Source: CAD feature listing. Evaluate the final solid. Frame: model axes, mm. A direction names the side the tool comes from. Give positions to 0.01 mm unless a question says otherwise; leave off trailing zeros. Order: outer loops, then holes, each group sorted by start corner. A loop starts at its lowest first (then second) coordinate and runs counter-clockwise, first axis right, second up.
1) Section A-A, the plane x = 0. Return loops of the section in (y, z), plus the area to 3 significant figures.
2) Section B-B, the plane z = 5. Return loops of the section in (x, y).
3) Draft query along Y for faces 3 (the face through (15.035, 38.636, 2.958)), 4 (the face through (2, 14, 6)), 5 (the face through (0, 11.5, 3)), 6 (the face through (15, 40, 3)). Return one class per face: released by +Y, released by -Y, zero draft, split by the parting line, or undercut.
4) Material intervals for line 1 (Y direction, x = 1, z = 3.25); line 2 (X direction, y = 14.5, z = 3.25); line 3 (Y direction, x = 0, z = 4.75), sorted ascending.
5) First-contact query: P1, Ø2, axis at x = 6, z = 8, coming from the +Y side; P2, Ø1.5, axis at y = 27.5, z = 8.5, coming from the +X side; P3, Ø4, axis at x = 6, y = 23, coming from the -Z side; P4, Ø6, axis at x = -8.5, y = 17, coming from the -Z side. Flat tips, straight axial feed; report the tip coordinate or a pass-through.
6) Section D-D, the plane z = 1. Return loops of the section in (x, y), plus the area to 3 significant figures.
7) Access query for faces 1 (the face through (0, 35, 0)), 2 (the face through (13, 37, 6)). Directions: +Z, -Z, +X, -X, +Y, -Y. A direction counts if a zero-diameter tool reaches every point of the face in a straight line with its end or side. Return the directions, or none.
8) Section C-C, the plane y = 14.5. Return loops of the section in (x, z).
```python
from build123d import *
from build123d.topology import SkipClean

# Parameters (mm, degrees)
SKICA1_R                            = 1.650000859
SKICA1_R_2                          = 1.650000856
SKICA1_R_3                          = 1.649999795
P_IDAT_VYSUNUT_M1_DEPTH             = 2
P_IDAT_VYSUNUT_M3_REACH             = 52.341
P_IDAT_VYSUNUT_M3_DIRECTION_2_REACH = 52.341
SKICA3_R                            = 7.749999856
ODEBRAT_VYSUNUT_M1_DEPTH            = 50
SKICA5_W                            = 5.707521684
SKICA5_H                            = 11.749115372
SKICA5_W_2                          = 4.565648586
ODEBRAT_VYSUNUT_M2_DEPTH            = 100
SKICA6_W                            = 8.00000038
SKICA6_H                            = 6.259476141
SKICA6_R                            = 1.649999795
SKICA6_W_2                          = 7.999999449
SKICA6_H_2                          = 6.147887642
SKICA6_R_2                          = 1.650000859
SKICA6_R_3                          = 1.650000856
P_IDAT_VYSUNUT_M4_DEPTH             = 4


with BuildPart() as part:
    # Skica1 → Přidat vysunutím1 (new body)
    with BuildSketch(Plane.XY):
        Polygon((19.249999896, 35.500001162), (19.249999896, 33.428542316), (4.00000019, 16.00000076), (4.00000019, 11.500000022), (-4.00000019, 11.500000022), (-4.00000019, 16.00000076), (-19.249999896, 33.42806357), (-19.249999896, 35.500001162), (-19.249999896, 39.999999106), (-11.250000447, 39.999999106), (-11.250000447, 35.500001162), (11.250000447, 35.500001162), (11.250000447, 39.999999106), (19.249999896, 39.999999106), align=None)
        with Locations((-15.249999503, 37.000001471)):
            Circle(SKICA1_R, mode=Mode.SUBTRACT)
        with Locations((15.249998879, 37.000001475)):
            Circle(SKICA1_R_2, mode=Mode.SUBTRACT)
        with Locations((1.87e-07, 14.499999779)):
            Circle(SKICA1_R_3, mode=Mode.SUBTRACT)
    extrude(amount=P_IDAT_VYSUNUT_M1_DEPTH)

    # Přidat vysunutím3: up to this face of the body (flat: up to its plane)
    p_idat_vysunut_m3_end = Plane(part.part.faces().sort_by_distance((11.625000043, 24.714271538, 1))[0])
    # Skica2 → Přidat vysunutím3 (add, up to the picked face)
    with BuildSketch(Plane(origin=(-11.250000447, 0, 0), x_dir=(0, 0, -1), z_dir=(1, 0, 0)), mode=Mode.PRIVATE) as p_idat_vysunut_m3_sk1:
        with BuildLine():
            Line((-2, 35.453607186), (-2, 33.44155343))
            ThreePointArc((-2, 33.44155343), (-8.800000314, 25.749999709), (-2, 18.058445988))
            Line((-2, 18.058445988), (-2, 16.046392232))
            ThreePointArc((-2, 16.046392232), (-10.800000314, 25.749999709), (-2, 35.453607186))
        make_face()
    p_idat_vysunut_m3_tool1 = split(extrude(p_idat_vysunut_m3_sk1.sketch, amount=P_IDAT_VYSUNUT_M3_REACH, mode=Mode.PRIVATE), bisect_by=p_idat_vysunut_m3_end, keep=Keep.BOTH, mode=Mode.PRIVATE)
    add(p_idat_vysunut_m3_tool1.solids().sort_by(Axis((-11.25, 17.052419, 2.213092), (1, 0, 0)))[0])

    # Přidat vysunutím3 direction 2: up to this face of the body (flat: up to its plane)
    p_idat_vysunut_m3_direction_2_end = Plane(part.part.faces().sort_by_distance((-11.625000043, 24.714032165, 1))[0])
    # Skica2 → Přidat vysunutím3 direction 2 (add, up to the picked face)
    with BuildSketch(Plane(origin=(-11.250000447, 0, 0), x_dir=(0, 0, -1), z_dir=(1, 0, 0)), mode=Mode.PRIVATE) as p_idat_vysunut_m3_direction_2_sk1:
        with BuildLine():
            Line((-2, 35.453607186), (-2, 33.44155343))
            ThreePointArc((-2, 33.44155343), (-8.800000314, 25.749999709), (-2, 18.058445988))
            Line((-2, 18.058445988), (-2, 16.046392232))
            ThreePointArc((-2, 16.046392232), (-10.800000314, 25.749999709), (-2, 35.453607186))
        make_face()
    p_idat_vysunut_m3_direction_2_tool1 = split(extrude(p_idat_vysunut_m3_direction_2_sk1.sketch, amount=-P_IDAT_VYSUNUT_M3_DIRECTION_2_REACH, mode=Mode.PRIVATE), bisect_by=p_idat_vysunut_m3_direction_2_end, keep=Keep.BOTH, mode=Mode.PRIVATE)
    add(p_idat_vysunut_m3_direction_2_tool1.solids().sort_by(Axis((-11.25, 17.052419, 2.213092), (-1, 0, 0)))[0])

    # Skica3 → Odebrat vysunutím1 (cut, symmetric)
    with SkipClean():  # the faces are left unmerged after this step: merging them gives an invalid solid
        with BuildSketch(Plane(origin=(-11.250000447, 0, 0), x_dir=(0, 0, -1), z_dir=(1, 0, 0))):
            with Locations((-1.050000457, 25.749999709)):
                Circle(SKICA3_R)
        extrude(amount=ODEBRAT_VYSUNUT_M1_DEPTH, both=True, mode=Mode.SUBTRACT)

    # Skica5 → Odebrat vysunutím2 (cut)
    with BuildSketch(Plane(origin=(0, 0, 0), x_dir=(-1, 0, 0), z_dir=(0, 0, -1))):
        Polygon((4.00000019, 16.00000076), (13.371125893, 26.709546366), (13.371125893, 14.106664416), align=None)
        with Locations((22.103760738, 34.12544142)):
            Rectangle(SKICA5_W, SKICA5_H)
        with Locations((-21.532824189, 34.12544142)):
            Rectangle(SKICA5_W_2, SKICA5_H)
    extrude(amount=-ODEBRAT_VYSUNUT_M2_DEPTH, mode=Mode.SUBTRACT)

    # Skica6 → Přidat vysunutím4 (add)
    # profile 1 of 3: a face of its own
    with BuildSketch(Plane.XY.offset(2)):
        with Locations((0, 14.629738093)):
            Rectangle(SKICA6_W, SKICA6_H)
        with Locations((1.87e-07, 14.499999779)):
            Circle(SKICA6_R, mode=Mode.SUBTRACT)
    # profile 2 of 3: a face of its own
    with BuildSketch(Plane.XY.offset(2)):
        with Locations((-15.250000172, 36.926055285)):
            Rectangle(SKICA6_W_2, SKICA6_H_2)
        with Locations((-15.249999503, 37.000001471)):
            Circle(SKICA6_R_2, mode=Mode.SUBTRACT)
    # profile 3 of 3: a face of its own
    with BuildSketch(Plane.XY.offset(2)):
        with Locations((15.250000172, 36.926055285)):
            Rectangle(SKICA6_W_2, SKICA6_H_2)
        with Locations((15.249998879, 37.000001475)):
            Circle(SKICA6_R_3, mode=Mode.SUBTRACT)
    extrude(amount=P_IDAT_VYSUNUT_M4_DEPTH)


solid = part.part
```
From the geometry:
1. outline: (11.5, 0) - (12.85, 0) - (12.85, 6) - (11.5, 6) - close; (16.05, 2) - (16.15, 2) - (16.15, 0) - (18.07, 0) arc R7.75 cw (long way) to (33.43, 0) - (35.5, 0) - (35.5, 2) - (35.45, 2) arc R9.75 ccw to (17.35, 6) - (16.15, 6) - (16.15, 2.75) arc R9.75 ccw to start
1. area: 68.6 mm2
2. outline: (-19.25, 33.43) - (-18.37, 32.42) - (18.37, 32.42) - (19.25, 33.43) - (19.25, 40) - (11.25, 40) - (11.25, 34.66) - (-11.25, 34.66) - (-11.25, 40) - (-19.25, 40) - close; (-6.7, 19.08) - (-4.73, 16.84) - (-4, 16.84) - (-4, 11.5) - (4, 11.5) - (4, 16.84) - (4.73, 16.84) - (6.7, 19.08) - close; hole circle Ø3.3 at (-15.25, 37); hole circle Ø3.3 at (0, 14.5); hole circle Ø3.3 at (15.25, 37)
3. face 3: undercut
3. face 4: zero draft
3. face 5: released by -Y
3. face 6: released by +Y
4. line 1: y = 11.5 to 13.19, 15.81 to 18.32, 33.18 to 35.25
4. line 2: x = -4 to -1.65, 1.65 to 4
4. line 3: y = 11.5 to 12.85, 16.15 to 18.94, 32.56 to 34.77
5. P1: stops at y = 33.47
5. P2: stops at x = 14.72
5. P3: stops at z = 7.17
5. P4: stops at z = 0
6. outline: (-19.25, 33.5) - (19.25, 33.5) - (19.25, 40) - (11.25, 40) - (11.25, 35.5) - (-11.25, 35.5) - (-11.25, 40) - (-19.25, 40) - close; (-5.75, 18) - (-4, 16) - (-4, 11.5) - (4, 11.5) - (4, 16) - (5.75, 18) - close; hole circle Ø3.3 at (-15.25, 37); hole circle Ø3.3 at (0, 14.5); hole circle Ø3.3 at (15.25, 37)
6. area: 179 mm2
7. face 1: -Z, +X, -X, +Y, -Y
7. face 2: +Z, +X, -X, +Y
8. outline: (-4, 0) - (-1.65, 0) - (-1.65, 6) - (-4, 6) - close; (1.65, 0) - (4, 0) - (4, 6) - (1.65, 6) - close
